from build123d import *

# Parameters (mm, degrees)
SKETCH1_R           = 9.525
BOSS_EXTRUDE1_DEPTH = 19.05
SKETCH2_R           = 6.35
BOSS_EXTRUDE2_DEPTH = 71.12
CUT_EXTRUDE1_DEPTH  = 9.144
CUT_EXTRUDE2_START  = -3.175
CUT_EXTRUDE2_DEPTH  = 12.7


with BuildPart() as part:
    # Sketch1 → Boss-Extrude1 (new body)
    with BuildSketch(Plane.XY):
        Circle(SKETCH1_R)
    extrude(amount=BOSS_EXTRUDE1_DEPTH)

    # Sketch2 → Boss-Extrude2 (add)
    with BuildSketch(Plane(origin=(0, 0, 0), x_dir=(-1, 0, 0), z_dir=(0, 0, -1))):
        with Locations(Location((0, 0, 0), (0, 0, 180))):  # turned: the seam where the file's is
            Circle(SKETCH2_R)
    extrude(amount=BOSS_EXTRUDE2_DEPTH)

    # Sketch3 → Cut-Extrude1 (cut)
    with BuildSketch(Plane(origin=(0, 0, -71.12), x_dir=(-1, 0, 0), z_dir=(0, 0, -1))):
        with BuildLine():
            Line((-1.277821972, 1.524), (1.277821972, 1.524))
            ThreePointArc((1.277821972, 1.524), (1.98882, 0), (1.277821972, -1.524))
            Line((1.277821972, -1.524), (-1.277821972, -1.524))
            ThreePointArc((-1.277821972, -1.524), (-1.98882, 0), (-1.277821972, 1.524))
        make_face()
    extrude(amount=-CUT_EXTRUDE1_DEPTH, mode=Mode.SUBTRACT)

    # Sketch4 → Cut-Extrude2 (cut)
    with BuildSketch(Plane.XY.offset(19.05).offset(CUT_EXTRUDE2_START)):
        with BuildLine():
            Line((0, 4.7625), (-1.308111225, 4.7625))
            Line((-1.308111225, 4.7625), (-4.019808446, 8.635204981))
            ThreePointArc((-4.019808446, 8.635204981), (0.004701224, 9.52499884), (4.028330588, 8.631232686))
            Line((4.028330588, 8.631232686), (1.319414798, 4.7625))
            Line((1.319414798, 4.7625), (0, 4.7625))
        make_face()
    extrude(amount=-CUT_EXTRUDE2_DEPTH, mode=Mode.SUBTRACT)


solid = part.part
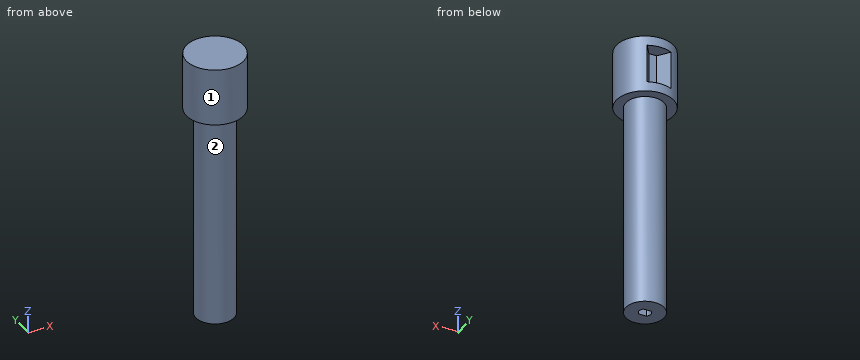
Could you check a few things on this model? Use its own coordinates, in mm. Face numbers are marked on the shaded views. A direction names the side the tool comes from. Round coordinates to 2 decimals unless told otherwise and drop trailing zeros. Order: outer loops, then holes, each group sorted by start corner. A loop starts at its lowest first (then second) coordinate and runs counter-clockwise, first axis right, second up. Notation, with made-up numbers: M 43,39 L 70,39 A24 cw 70,72 Z; hole C -10,21 d2. An arc over 180 degrees is marked long. One line per item, written item: value.
(1) Which directions (+Z, -Z, +X, -X, +Y, -Y) give clear straight access to the entire face, cutting with the end or side of a thin tool? Please do the marked faces 1 and 2.
Ans:
face 1: +Z, -Z
face 2: -Z
(2) I'm going to push flat-ended pins straight in: P1, Ø1, axis at x = 4.5, z = -27.5, coming from the +Y side; P2, Ø5, axis at x = -6.5, z = -1.5, coming from the -Y side (3 decimals); P3, Ø8, axis at x = -1, z = -38, coming from the -Y side; P4, Ø4, axis at x = 1, y = 8, coming from the -Z side. Where does each tip first touch, or does it pass through?
Ans:
P1: stops at y = 4.93
P2: stops at y = -8.395
P3: stops at y = -6.35
P4: stops at z = -71.12
(3) I need wall thicknesses on line 1 along Z through (x, y) = (-0.75, 6) (3 decimals); line 2 along Z through (x, y) = (8.75, -3); line 3 along Y through (x, z) = (0.25, -61.5). Which ranges of each line are inside material? Lowest first, please. Write a range as from..to.
Ans:
line 1: z = -71.12..3.175, 15.875..19.05
line 2: z = 0..19.05
line 3: y = -6.35..6.35
(4) Imagine slicing it at C-C (y = 7.25). Write out the boundary of the cut face in (x, z) (3 decimals), and give its area (3 significant figures).
Ans:
outline: M -6.178,0 L 6.178,0 L 6.178,19.05 L -6.178,19.05 Z; hole M -3.05,3.175 L 3.061,3.175 L 3.061,15.875 L -3.05,15.875 Z
area: 158 mm^2
(5) Imagine slicing it at B-B (y = 0). Write out the boundary of the cut face in (x, z) (3 decimals).
Ans:
outline: M -9.525,0 L -6.35,0 L -6.35,-71.12 L -1.989,-71.12 L -1.989,-61.976 L 1.989,-61.976 L 1.989,-71.12 L 6.35,-71.12 L 6.35,0 L 9.525,0 L 9.525,19.05 L -9.525,19.05 Z
